Study the drawing (mm; zero at the part's minimum x, y, z) and answer. A direction names the side the tool comes from. Coordinates: 2 decimals unless noted, no trailing zeros. Loops run counter-clockwise (first coordinate to the right, second up) from the corner with the lowest first, then second, coordinate; pieces in that order, holes last. Notation, with made-up numbers: (-7.5, 66.25) - (13.5, 66.25) arc R19 ccw to (13.5, 99.25) - close; hole circle Ø2 at (35.25, 86). An arc over 180 degrees is marked (long way). Put each result on its own line as item: value.
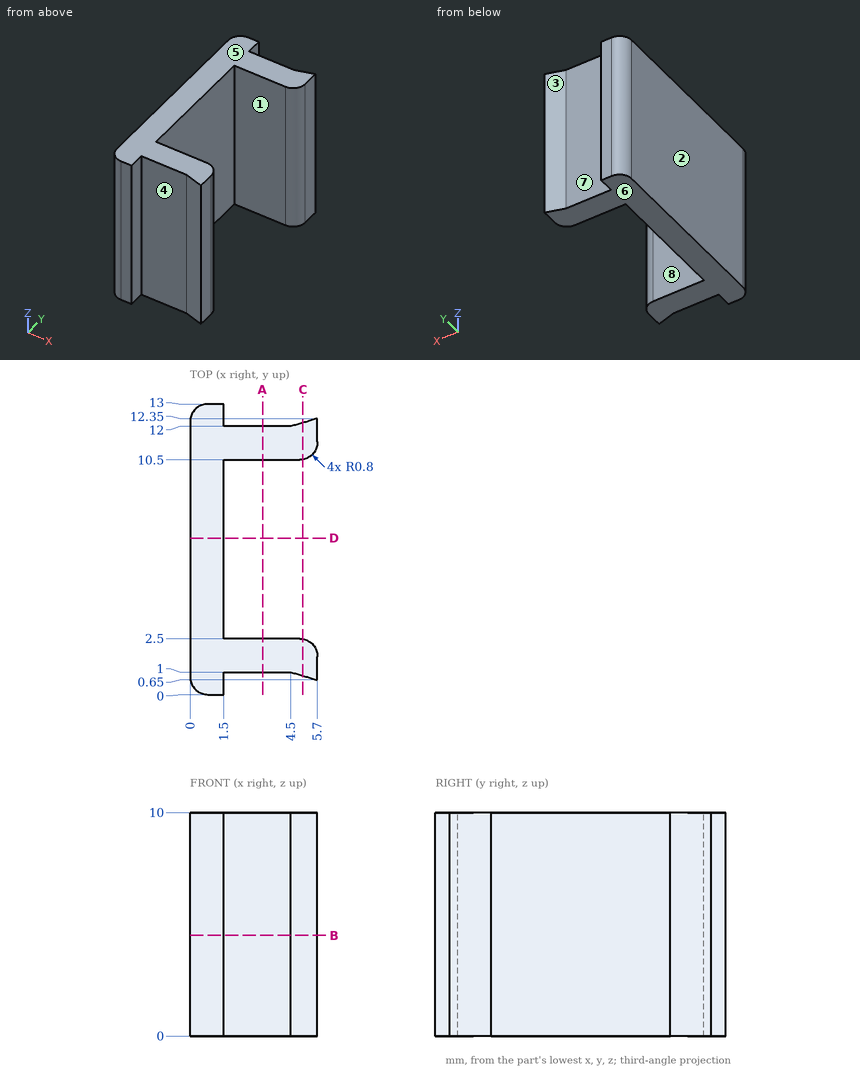
1) For a pull along Y with two mould halves and no side action, classify the marked faces 6, 7 and 8 as pulls with the +Y half, pulls with the -Y half, needs draft (parallel to the pull), parting line crosses it, or undercut.
Found:
face 6: needs draft
face 7: pulls with the +Y half
face 8: undercut
2) Each of these flat-tipped pins is pushed along its axis until it touches: pin 1 (2.5 mm diameter, centred on y = 6, z = 3.5, fed in from +X); pin 2 (1 mm diameter, centred on x = 4.5, z = 1, fed in from +Y); pin 3 (2.5 mm diameter, centred on x = 3, z = 5.5, fed in from -Y). Where does it stop, or does it pass through?
Found:
pin 1: stops at x = 1.5
pin 2: stops at y = 12.15
pin 3: stops at y = 1
3) The part is cut by section D-D (y = 7). Give the vertices of the cut face in (x, z), and give its area (3 significant figures).
Found:
outline: (0, 0) - (1.5, 0) - (1.5, 10) - (0, 10) - close
area: 15.0 mm^2
4) For the marked faces 1, 2, 3, 4 and 5, determine the directions among +Z, -Z, +X, -X, +Y, -Y from which every point of the face is accessible in a straight line to the end or side of a thin tool.
Found:
face 1: +Z, -Z, +X
face 2: +Z, -Z, -X, +Y, -Y
face 3: +Z, -Z, +Y
face 4: +Z, -Z, -Y
face 5: +Z, +X, -X, +Y, -Y
5) The part is cut by section C-C (x = 5.05). Give the vertices of the cut face in (y, z).
Found:
outline: (0.84, 0) - (2.49, 0) - (2.49, 10) - (0.84, 10) - close; (10.51, 0) - (12.16, 0) - (12.16, 10) - (10.51, 10) - close
6) The part is cut by section B-B (z = 4.5). Give the vertices of the cut face in (x, y).
Found:
outline: (0, 0.8) arc R0.8 ccw to (0.8, 0) - (1.5, 0) - (1.5, 1) - (4.5, 1) - (5.7, 0.65) - (5.7, 1.7) arc R0.8 ccw to (4.9, 2.5) - (1.5, 2.5) - (1.5, 10.5) - (4.9, 10.5) arc R0.8 ccw to (5.7, 11.3) - (5.7, 12.35) - (4.5, 12) - (1.5, 12) - (1.5, 13) - (0.8, 13) arc R0.8 ccw to (0, 12.2) - close
7) The part is cut by section A-A (x = 3.25). Give the vertices of the cut face in (y, z).
Found:
outline: (1, 0) - (2.5, 0) - (2.5, 10) - (1, 10) - close; (10.5, 0) - (12, 0) - (12, 10) - (10.5, 10) - close
8) Straight lines are drawn through the part: L1, parallel to Y at x = 3.3, z = 2; L2, parallel to X at y = 7.5, z = 9; L3, parallel to X at y = 0.5, z = 8.5. For each, find the intervals that lie inside material, in ascending order. Write a range as [from, to].
Found:
L1: y = [1, 2.5], [10.5, 12]
L2: x = [0, 1.5]
L3: x = [0.06, 1.5]
